Verification items for the finished model (mm, model axes). A direction names the side the tool comes from. Round coordinates to 2 decimals unless told otherwise and drop trailing zeros. Write each loop counter-clockwise with the first axis right and the second up, starting at its lowest first coordinate (ties: lowest second). Pieces come first, ordered by that corner, then holes. Notation, with made-up numbers: M -9.75,32 L 36.25,32 A13 cw 36.25,40 Z; hole C -5.5,-9.75 d1. An arc over 180 degrees is marked long. Answer in a Markdown table with one row per item. Add a question column.
1. Set-up check for faces 4 (the flat face through (31, 22.428, 12)), 5 (the flat face through (32, 1, 5)), 6 (the flat face through (32, 2.829, 4)): record each of +Z, -Z, +X, -X, +Y, -Y from which the full face is reachable in a straight line by a thin tool's end or side.
2. Sectioned sample at D-D on x = 38.25. Record the cut outline in (y, z), plus the area to 3 significant figures.
3. Sectioned sample at C-C on y = 9. Record the cut outline in (x, z), plus the area to 3 significant figures.
4. Sectioned sample at B-B on z = 6.25. Record the cut outline in (x, y), plus the area to 3 significant figures.
5. Sectioned sample at A-A on x = 35. Record the cut outline in (y, z).
6. Go/stop test with a flat-tipped pin: pin 1 Ø3.5 at (x, z) = (31, 5) entering from +Y. Record where the tip stops, or that it passes through.
7. Draft check along Z on faces 1 (the flat face through (42.133, 15, 6)), 2 (the flat face through (35.633, 1, 8)), 3 (the flat face through (31, 11, 15)). Enter one of: pulls with the +Z half, pulls with the -Z half, needs draft (parallel to the pull), parting line crosses it, or undercut.
8. Material ranges on probe 1 along Z at (x, y) = (34, 14.5); probe 2 along X at (y, z) = (18, 4); probe 3 along Y at (x, z) = (23.5, 10.75), recorded low to high.
Autodesk Inventor part; units mm, degrees
ref_plane "YZ Plane" through (0, 0, 0) normal (1, 0, 0) x (0, 1, 0)
ref_plane "XZ Plane" through (0, 0, 0) normal (0, 1, 0) x (-1, 0, 0)
ref_plane "XY Plane" through (0, 0, 0) normal (0, 0, 1) x (1, 0, 0)
sketch "Sketch1" plane through (0, 0, 0) normal (0, 0, 1) x (1, 0, 0)
  line L0 (24.1334, 37.8287) -> (39.1334, 37.8287)
  line L1 (39.1334, 37.8287) -> (39.1334, 2.8287)
  line L2 (39.1334, 2.8287) -> (24.1334, 2.8287)
  line L3 (24.1334, 2.8287) -> (24.1334, 37.8287)
  line L4 (42.1334, 40.8287) -> (21.1334, 40.8287)
  line L5 (21.1334, 40.8287) -> (21.1334, -0.1713)
  line L6 (21.1334, -0.1713) -> (42.1334, -0.1713)
  line L7 (42.1334, -0.1713) -> (42.1334, 40.8287)
  line L8 (21.1334, 22.4276) -> (42.1334, 22.4276)
  point P0 (0, 0)
  point P1 (24.1334, 22.4276)
  point P2 (39.1334, 22.4276)
  dimension "d0" = 15
  dimension "d1" = 35
  dimension "d2" = 3
extrude "Extrusion1" add sketch "Sketch1" along normal blind 3
extrude "Extrusion2" add sketch "Sketch1" along normal blind 15 contours L3 L2 L1 L8 L7 L6 L5
extrude "Extrusion3" add sketch "Sketch1" along normal blind 15 contours L8 L1 L2 L3
extrude "Extrusion4" cut sketch "Sketch1" along normal blind 10 contours L8 L1 L2 L3
extrude "Extrusion5" add sketch "Sketch1" along normal blind 3 contours L8 L1 L2 L3
sketch "Sketch2" plane through (24.1334, 2.8287, 3) normal (0, 1, 0) x (1, 0, 0)
  line L0 (0, -7) -> (15, -7)
  line L1 (3.5, -7) -> (11.5, -7)
  line L2 (11.5, -7) -> (11.5, -2)
  line L3 (11.5, -2) -> (3.5, -2)
  line L4 (3.5, -2) -> (3.5, -7)
  line L5 (0, -7) -> (0, 0)
  point P0 (-24.1334, 3)
  dimension "d13" = 8
  dimension "d14" = 5
  dimension "d15" = 3.5
extrude "Extrusion6" cut sketch "Sketch2" against normal blind 3
properties part number "IRsensorhub"
Geometry check:
| question | item | result |
|---|---|---|
| 1 | face 4 | +Z, +X, -X, +Y |
| 1 | face 5 | +Y, -Y |
| 1 | face 6 | +Y |
| 2 | outline | M -0.17,0 L 40.83,0 L 40.83,3 L 2.83,3 L 2.83,10 L 22.43,10 L 22.43,15 L -0.17,15 Z |
| 2 | area | 257 mm2 |
| 3 | outline | M 21.13,0 L 42.13,0 L 42.13,15 L 21.13,15 Z; hole M 24.13,3 L 39.13,3 L 39.13,10 L 24.13,10 Z |
| 3 | area | 210 mm2 |
| 4 | outline | M 21.13,-0.17 L 27.63,-0.17 L 27.63,2.83 L 24.13,2.83 L 24.13,22.43 L 21.13,22.43 Z; M 35.63,-0.17 L 42.13,-0.17 L 42.13,22.43 L 39.13,22.43 L 39.13,2.83 L 35.63,2.83 Z |
| 4 | area | 157 mm2 |
| 5 | outline | M -0.17,0 L 40.83,0 L 40.83,3 L 2.83,3 L 2.83,5 L -0.17,5 Z; M -0.17,10 L 22.43,10 L 22.43,15 L -0.17,15 Z |
| 6 | pin 1 | stops at y = 2.83 |
| 7 | face 1 | needs draft |
| 7 | face 2 | undercut |
| 7 | face 3 | pulls with the +Z half |
| 8 | probe 1 | z = 0 to 3, 10 to 15 |
| 8 | probe 2 | x = 21.13 to 24.13, 39.13 to 42.13 |
| 8 | probe 3 | y = -0.17 to 22.43 |
